from build123d import *

# Parameters (mm, degrees)
BOSS_EXTRUDE1_DEPTH = 225
BOSS_EXTRUDE2_DEPTH = 10
SKETCH6_W           = 210
SKETCH6_H           = 200
BOSS_EXTRUDE3_DEPTH = 15
SKETCH5_R           = 2.1
CUT_EXTRUDE1_DEPTH  = 4.5
SKETCH10_W          = 210
SKETCH10_H          = 200
BOSS_EXTRUDE4_DEPTH = 40
SKETCH11_R          = 5
BOSS_EXTRUDE5_DEPTH = 5
BOSS_EXTRUDE5_TAPER = 5
SKETCH13_W          = 185
SKETCH13_H          = 10
BOSS_EXTRUDE6_DEPTH = 47.5
SKETCH14_W          = 185
SKETCH14_H          = 10
BOSS_EXTRUDE7_DEPTH = 47.5
SKETCH7_W           = 21
SKETCH7_H           = 10.25
CUT_EXTRUDE2_DEPTH  = 15
SKETCH15_R          = 2.1
CUT_EXTRUDE4_DEPTH  = 4.5
FILLET2_R           = 10
FILLET4_R           = 5


with BuildPart() as part:
    # Sketch2 → Boss-Extrude1 (new body)
    with BuildSketch(Plane(origin=(0, 0, 0), x_dir=(1, 0, 0), z_dir=(0, 1, 0))):
        Polygon((-90, 0), (90, 0), (90, -185), (105, -185), (105, 15), (-105, 15), (-105, -185), (-90, -185), align=None)
    extrude(amount=BOSS_EXTRUDE1_DEPTH)

    # Sketch3 → Boss-Extrude2 (add)
    with BuildSketch(Plane(origin=(0, 10, 0), x_dir=(1, 0, 0), z_dir=(0, 1, 0))):
        Polygon((-90, -185), (-22.5, -185), (-22.5, -10), (22.5, -10), (22.5, -185), (90, -185), (90, 0), (-90, 0), align=None)
    extrude(amount=BOSS_EXTRUDE2_DEPTH)

    # Sketch6 → Boss-Extrude3 (add)
    with BuildSketch(Plane.XZ):
        with Locations((0, 85)):
            Rectangle(SKETCH6_W, SKETCH6_H)
    extrude(amount=BOSS_EXTRUDE3_DEPTH)

    # Sketch5 → Cut-Extrude1 (cut)
    with BuildSketch(Plane.XY.offset(185)):
        with Locations((-97.5, 217.5)):
            Circle(SKETCH5_R)
        with Locations((97.5, 217.5)):
            Circle(SKETCH5_R)
        with Locations((-97.5, -7.5)):
            Circle(SKETCH5_R)
        with Locations((97.5, -7.5)):
            Circle(SKETCH5_R)
    extrude(amount=-CUT_EXTRUDE1_DEPTH, mode=Mode.SUBTRACT)

    # Sketch10 → Boss-Extrude4 (add)
    with BuildSketch(Plane.XZ.offset(15)):
        with Locations((0, 85)):
            Rectangle(SKETCH10_W, SKETCH10_H)
    extrude(amount=BOSS_EXTRUDE4_DEPTH)

    # Sketch11 → Boss-Extrude5 (add)
    with BuildSketch(Plane(origin=(0, 0, 0), x_dir=(1, 0, 0), z_dir=(0, 1, 0))):
        with Locations((0, -90)):
            Circle(SKETCH11_R)
    extrude(amount=BOSS_EXTRUDE5_DEPTH, taper=BOSS_EXTRUDE5_TAPER)

    # Sketch13 → Boss-Extrude6 (add)
    with BuildSketch(Plane.ZY.offset(-90)):
        with Locations((92.5, 5)):
            Rectangle(SKETCH13_W, SKETCH13_H)
    extrude(amount=BOSS_EXTRUDE6_DEPTH)

    # Sketch14 → Boss-Extrude7 (add)
    with BuildSketch(Plane(origin=(-90, 0, 0), x_dir=(0, 0, -1), z_dir=(1, 0, 0))):
        with Locations((-92.5, 5)):
            Rectangle(SKETCH14_W, SKETCH14_H)
    extrude(amount=BOSS_EXTRUDE7_DEPTH)

    # Sketch7 → Cut-Extrude2 (cut)
    with BuildSketch(Plane(origin=(0, 0, -15), x_dir=(-1, 0, 0), z_dir=(0, 0, -1))):
        with Locations((-32, 5.125)):
            Rectangle(SKETCH7_W, SKETCH7_H)
    extrude(amount=-CUT_EXTRUDE2_DEPTH, mode=Mode.SUBTRACT)

    # Sketch15 → Cut-Extrude4 (cut)
    with BuildSketch(Plane(origin=(0, 225, 0), x_dir=(1, 0, 0), z_dir=(0, 1, 0))):
        with Locations((0, 7.5)):
            Circle(SKETCH15_R)
        with Locations((-97.5, -90)):
            Circle(SKETCH15_R)
        with Locations((97.5, -90)):
            Circle(SKETCH15_R)
    extrude(amount=-CUT_EXTRUDE4_DEPTH, mode=Mode.SUBTRACT)

    # Fillet2
    fillet2_edges = [part.edges().sort_by_distance(p)[0] for p in [
        (90, 122.5, 0),
        (-90, 122.5, 0),
    ]]
    fillet(fillet2_edges, radius=FILLET2_R)

    # Fillet4
    fillet4_edges = [part.edges().sort_by_distance(p)[0] for p in [
        (-105, 85, -15),
        (105, 85, -15),
    ]]
    fillet(fillet4_edges, radius=FILLET4_R)


solid = part.part
Could you check a few things on this model? Use its own coordinates, in mm. A direction names the side the tool comes from. Round coordinates to 2 decimals unless told otherwise and drop trailing zeros. Order: outer loops, then holes, each group sorted by start corner. A loop starts at its lowest first (then second) coordinate and runs counter-clockwise, first axis right, second up. Notation, with made-up numbers: M 52.25,-10.75 L 65.25,-10.75 A12 ccw 65.25,-1.75 Z; hole C 19.5,-10 d8. An arc over 180 degrees is marked long. One line per item, written item: value.
(1) Imagine slicing it at C-C (z = 57). Write out the boundary of the cut face in (x, y), and give its area (3 significant figures).
Ans:
outline: M -105,-55 L 105,-55 L 105,225 L 90,225 L 90,20 L 22.5,20 L 22.5,10 L 42.5,10 L 42.5,0 L -42.5,0 L -42.5,10 L -22.5,10 L -22.5,20 L -90,20 L -90,225 L -105,225 Z
area: 20,600 mm^2
(2) Imagine slicing it at B-B (y = 27). Write out the boundary of the cut face in (x, z), and give its area (3 significant figures).
Ans:
outline: M -105,-10 A5 ccw -100,-15 L 100,-15 A5 ccw 105,-10 L 105,185 L 90,185 L 90,10 A10 cw 80,0 L -80,0 A10 cw -90,10 L -90,185 L -105,185 Z
area: 8,730 mm^2
(3) If we mould it in two halves opening along X, with no side actions, what happens to faces 1 (the flat face through (-1, -10, 185)), 2 (the flat face through (-105, 87, 86)), 3 (the flat face through (9, 0, 86))? For each: released by +X, released by -X, zero draft, split by the parting line, or undercut.
Ans:
face 1: zero draft
face 2: released by -X
face 3: undercut
(4) I'm going to push flat-ended pins straight in: P1, Ø1, axis at x = 35, y = 41.5, coming from the +Z side; P2, Ø3.5, axis at x = -97.5, y = 217.5, coming from the +Z side; P3, Ø1, axis at x = 58.5, z = 120, coming from the +Y side. Where does each tip first touch, or does it pass through?
Ans:
P1: stops at z = 0
P2: stops at z = 180.5
P3: stops at y = 20
(5) Which directions (+Z, -Z, +X, -X, +Y, -Y) give clear straight access to the entire face, cutting with the end or side of a thin tool? Please do faces 4 (the cylindrical face through (-87.15, 123.94, 3.01)), 5 (the flat face through (105, 87, 86)), 6 (the flat face through (-42.5, 5, 94)), 7 (the flat face through (32, 10.25, -8)).
Ans:
face 4: +Z, +Y
face 5: +Z, -Z, +X, +Y, -Y
face 6: +Z
face 7: -Z
(6) Imagine slicing it at A-A (x = 14). Write out the boundary of the cut face in (y, z), and give its area (3 significant figures).
Ans:
outline: M -55,-15 L 225,-15 L 225,0 L 20,0 L 20,10 L 10,10 L 10,0 L 0,0 L 0,185 L -55,185 Z
area: 14,500 mm^2
(7) Imagine slicing it at D-D (x = -34). Write out the boundary of the cut face in (y, z), and give its area (3 significant figures).
Ans:
outline: M -55,-15 L 225,-15 L 225,0 L 20,0 L 20,185 L 10,185 L 10,0 L 0,0 L 0,185 L -55,185 Z
area: 16,200 mm^2
(8) I need wall thicknesses on line 1 along Y through (x, z) = (97.5, 181.4); line 2 along X through (y, z) = (217.5, 182.9); line 3 along Z through (x, y) = (-97.5, 222.9). Which ranges of each line are inside material? Lowest first, please. Write a range as from..to.
Ans:
line 1: y = -55..-9.6, -5.4..215.4, 219.6..225
line 2: x = -105..-99.6, -95.4..-90, 90..95.4, 99.6..105
line 3: z = -15..87.9, 92.1..185
